Geometry: final body of the model. Coordinates: model frame, mm. A direction names the side the tool comes from. Give positions to 0.01 mm unless a question says otherwise; leave off trailing zeros. Loops run counter-clockwise (first coordinate to the right, second up) from the corner with the lowest first, then second, coordinate; pieces in that order, holes last. Notation, with made-up numbers: (-32.5, 47.25) -> (-19.5, 47.25) arc R27 cw to (-19.5, 77.25) -> close; hole circle Ø6 at (1.25, -34.75). An arc over 180 degrees is marked (long way). Answer in a Markdown table with one row per item. Add a question column.
Autodesk Inventor part; units mm, degrees
ref_plane "YZ Plane" through (0, 0, 0) normal (1, 0, 0) x (0, 1, 0)
ref_plane "XZ Plane" through (0, 0, 0) normal (0, 1, 0) x (-1, 0, 0)
ref_plane "XY Plane" through (0, 0, 0) normal (0, 0, 1) x (1, 0, 0)
sketch "Sketch1" plane through (0, 0, 0) normal (0, 1, 0) x (-1, 0, 0)
  line L0 (19, 13.208) -> (-19, 13.208)
  line L1 (-19, 13.208) -> (-19, -13.208)
  line L2 (-19, -13.208) -> (19, -13.208)
  line L3 (19, -13.208) -> (19, 13.208)
  line L4 (19, 13.208) -> (-19, -13.208) construction
  line L5 (-19, 13.208) -> (19, -13.208) construction
  circle A0 centre (16, -10.208) radius 1.75
  circle A1 centre (-16, 10.208) radius 1.75
  circle A2 centre (11.428, -5.518) radius 0.5
  circle A3 centre (8.888, -5.518) radius 0.5
  circle A4 centre (6.348, -5.518) radius 0.5
  circle A5 centre (3.808, -5.518) radius 0.5
  circle A6 centre (1.268, -5.518) radius 0.5
  line L6 (12.698, -6.788) -> (-0.002, -6.788)
  line L7 (-0.002, -6.788) -> (-0.002, -4.248)
  line L8 (-0.002, -4.248) -> (12.698, -4.248)
  line L9 (12.698, -4.248) -> (12.698, -6.788)
  circle A7 centre (-9.908, -5.518) radius 0.5
  circle A8 centre (-12.448, -5.518) radius 0.5
  circle A9 centre (-14.988, -5.518) radius 0.5
  line L10 (-8.638, -6.788) -> (-16.258, -6.788)
  line L11 (-16.258, -6.788) -> (-16.258, -4.248)
  line L12 (-16.258, -4.248) -> (-8.638, -4.248)
  line L13 (-8.638, -4.248) -> (-8.638, -6.788)
  line L14 (1.5071, -0.508) -> (-8.4529, -0.508)
  line L15 (-8.4529, -0.508) -> (-8.4529, 11.152)
  line L16 (-8.4529, 11.152) -> (1.5071, 11.152)
  line L17 (1.5071, 11.152) -> (1.5071, -0.508)
  point P0 (0, 0)
  dimension "d0" = 38
  dimension "d1" = 26.416
  dimension "d2" = 3.5
  dimension "d3" = 3.5
  dimension "d4" = 3
  dimension "d5" = 3
  dimension "d6" = 3
  dimension "d7" = 3
  dimension "d8" = 1
  dimension "d9" = 4.572
  dimension "d10" = 4.69
  dimension "d13" = 2.54
  dimension "d18" = 1.27
  dimension "d19" = 1.27
  dimension "d20" = 1.27
  dimension "d21" = 1.27
  dimension "d22" = 1
  dimension "d23" = 11.176
  dimension "d26" = 2.54
  dimension "d31" = 1.27
  dimension "d33" = 1.27
  dimension "d34" = 9.96
  dimension "d35" = 11.66
  dimension "d36" = 3.74
extrude "Extrusion1" add sketch "Sketch1" along normal blind 1.7 contours L3 L2 L1 L0
extrude "Extrusion2" add sketch "Sketch1" along normal blind 8.62 contours L14 L15 L16 L17
extrude "Extrusion3" add sketch "Sketch1" along normal blind 4.1 contours L6 L7 L8 L9 | L10 L11 L12 L13
sketch "Sketch2" plane through (19, 0, 13.208) normal (1, 0, 0) x (0, 0, -1)
  line L0 (18.9857, 6.15) -> (26.8557, 6.15)
  line L1 (0, 0) -> (26.416, 0)
  line L2 (18.9857, 6.15) -> (18.9857, 0)
  point P0 (13.208, 0)
  dimension "d43" = 6.15
  dimension "d44" = 7.87
sweep "Sweep1" add profiles "Sketch1" path "Sketch2" path curves L2 L0 contours A2 | A3 | A4 | A5 | A6 | A7 | A8 | A9
sketch "Sketch3" plane through (0, 1.7, 0) normal (0, 1, 0) x (1, 0, 0)
  line L0 (-13.5449, 4.016) -> (19.3166, 4.016) construction
  line L1 (19.3166, 4.016) -> (19.3166, 0.2862) construction
  line L2 (19.3166, 0.2862) -> (-13.5449, 0.2862) construction
  line L3 (-13.5449, 0.2862) -> (-13.5449, 4.016) construction
  point P0 (0, 0)
properties part number "modestmard"
(1) Cut plane B-B on y = 3.5. Return the cut outline in (x, z), then the cut area to 3 significant figures.
(2) Cut plane D-D on x = 11.5. Return the cut outline in (y, z), then the cut area to 3 significant figures.
(3) Cut plane A-A on x = -16. Return the cut outline in (y, z).
(4) Material intervals for line 1 along Z through (x, y) = (16, 0.75); line 2 along Z through (x, y) = (-16, 0.4); line 3 along X through (y, z) = (7, 8.5), sorted ascending. Write a range as from..to.
(5) Cut plane C-C on z = -11.5. State how many separate pieces and enclosed holes the cut face has, then the cut area to 3 significant figures.
(6) Reachability of faces 1 (the cylindrical face through (-6.579, 5.173, -5.074)), 2 (the flat face through (-12.698, 3, -6)), 3 (the flat face through (-6, 3, -6.788)), 4 (the cylindrical face through (-11.32, 6.898, -9.272)) from +Z, -Z, +X, -X, +Y, -Y: full face, straight path, thin tool, end or side. Return the list, or none.
(7) Pin query (flat end, axial travel): pin 1 Ø1 at (y, z) = (4, 3.5) entering from -X; pin 2 Ø0.7 at (x, y) = (-4, 2.5) entering from -Z; pin 3 Ø1.2 at (y, z) = (3, -6) entering from -X; pin 4 Ø3 at (x, z) = (-16, -10.208) entering from -Y. Return the tip coordinate at first contact, or that it passes through.
(8) Draft query along Y for faces 5 (the flat face through (12.5, 6.4, -13.648)), 6 (the cylindrical face through (-4.039, 5.173, -5.074)), 7 (the flat face through (0, 0, 0)). Return one class per face: +Y half, -Y half, draft (parallel to the pull), parting line (faces both ways), or undercut.
Answer list:
| question | item | result |
|---|---|---|
| 1 | outline | (-12.7, -6.79) -> (0, -6.79) -> (0, -4.25) -> (-12.7, -4.25) -> close; (-1.51, -0.51) -> (8.45, -0.51) -> (8.45, 11.15) -> (-1.51, 11.15) -> close; (8.64, -6.79) -> (16.26, -6.79) -> (16.26, -4.25) -> (8.64, -4.25) -> close |
| 1 | area | 168 mm² |
| 2 | outline | (0, -13.21) -> (1.7, -13.21) -> (1.7, -6.79) -> (4.1, -6.79) -> (4.1, -4.25) -> (1.7, -4.25) -> (1.7, 13.21) -> (0, 13.21) -> close |
| 2 | area | 51.0 mm² |
| 3 | outline | (0, -13.21) -> (1.7, -13.21) -> (1.7, -11.96) -> (0, -11.96) -> close; (0, -8.46) -> (1.7, -8.46) -> (1.7, 13.21) -> (0, 13.21) -> close |
| 4 | line 1 | z = -13.21..8.46, 11.96..13.21 |
| 4 | line 2 | z = -13.21..-11.96, -8.46..13.21 |
| 4 | line 3 | x = -1.51..8.45 |
| 5 | separate pieces | 10 |
| 5 | enclosed holes | 0 |
| 5 | area | 66.9 mm² |
| 6 | face 1 | none |
| 6 | face 2 | +Z, -Z, -X, +Y |
| 6 | face 3 | -Z, +X, -X |
| 6 | face 4 | -Z |
| 7 | pin 1 | stops at x = -1.51 |
| 7 | pin 2 | stops at z = -6.79 |
| 7 | pin 3 | stops at x = -12.7 |
| 7 | pin 4 | passes through |
| 8 | face 5 | draft |
| 8 | face 6 | undercut |
| 8 | face 7 | -Y half |
